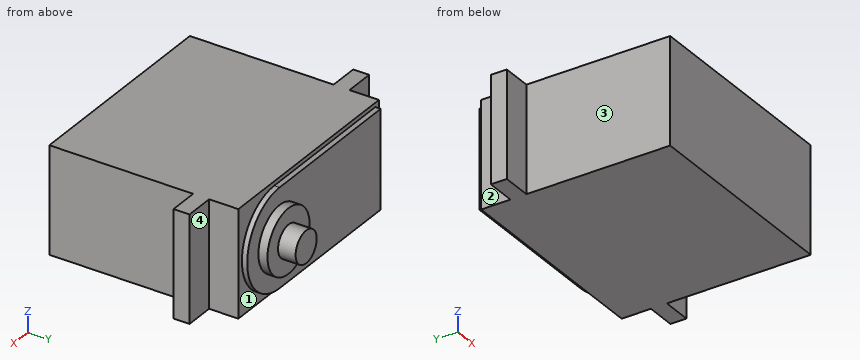
from build123d import *

# Parameters (mm, degrees)
RESSALTO_EXTRUS_O1_DEPTH = 10
RESSALTO_EXTRUS_O2_DEPTH = 1
ESBO_O4_R                = 3
RESSALTO_EXTRUS_O3_DEPTH = 5
ESBO_O5_R                = 6
RESSALTO_EXTRUS_O4_DEPTH = 1.7


with BuildPart() as part:
    # Esboço1 → Ressalto-extrusão1 (new body, symmetric)
    with BuildSketch(Plane.XY):
        Polygon((20, -0.767915455), (25.568877633, -0.767915455), (25.568877633, -3.767915455), (20, -3.767915455), (20, -30.767915455), (-20, -30.767915455), (-20, -3.767915455), (-25.568877633, -3.767915455), (-25.568877633, -0.767915455), (-20, -0.767915455), (-20, 4.732084545), (20, 4.732084545), align=None)
    extrude(amount=RESSALTO_EXTRUS_O1_DEPTH, both=True)

    # Esboço3 → Ressalto-extrusão2 (add)
    with BuildSketch(Plane(origin=(0, 4.732084545, 0), x_dir=(1, 0, 0), z_dir=(0, 1, 0))):
        with BuildLine():
            Line((-19, 9.2), (9.8, 9.2))
            ThreePointArc((9.8, 9.2), (19, 0), (9.8, -9.2))
            Line((9.8, -9.2), (-19, -9.2))
            Line((-19, -9.2), (-19, 9.2))
        make_face()
    extrude(amount=RESSALTO_EXTRUS_O2_DEPTH)

    # Esboço4 → Ressalto-extrusão3 (add)
    with BuildSketch(Plane(origin=(0, 5.732084545, 0), x_dir=(1, 0, 0), z_dir=(0, 1, 0))):
        with Locations((9.8, 0)):
            Circle(ESBO_O4_R)
    extrude(amount=RESSALTO_EXTRUS_O3_DEPTH)

    # Esboço5 → Ressalto-extrusão4 (add)
    with BuildSketch(Plane(origin=(0, 5.732084545, 0), x_dir=(1, 0, 0), z_dir=(0, 1, 0))):
        with Locations((9.8, 0)):
            Circle(ESBO_O5_R)
    extrude(amount=RESSALTO_EXTRUS_O4_DEPTH)


solid = part.part
Could you check a few things on this model? Use its own coordinates, in mm. Face numbers are marked on the shaded views. A direction names the side the tool comes from. Give positions to 0.01 mm unless a question says otherwise; leave off trailing zeros. Order: outer loops, then holes, each group sorted by start corner. A loop starts at its lowest first (then second) coordinate and runs counter-clockwise, first axis right, second up.
1. Will these pins go through, and if not, where does the flat tip stop? P1, Ø10, axis at x = -8, z = -2.5, coming from the +Y side; P2, Ø0.5, axis at x = -3.5, y = 5.5, coming from the +Z side; P3, Ø6, axis at y = 3, z = 0.5, coming from the -X side.
2. I need wall thicknesses on L1, parallel to Y at x = 2, z = 8.5; L2, parallel to X at y = -8, z = 6; L3, parallel to Y at x = 10, z = -3.5. Which ranges of each line are inside material? Lowest first, please.
3. Suppose I cut it at D-D (z = -7). List the corners of the cut face in (x, y) for me, plus the area to 3 significant figures.
4. Suppose I cut it at C-C (y = -27). List the corners of the cut face in (x, z) for me, plus the area to 3 significant figures.
5. Suppose I cut it at A-A (z = 0). List the corners of the cut face in (x, y) for me, plus the area to 3 significant figures.
6. For the marked faces 1, 2, 3 and 4, which set-ups out of +Z, -Z, +X, -X, +Y, -Y let a thin tool reach every point of the face, with its end or its side?
7. Suppose I cut it at B-B (x = -14.5). List the corners of the cut face in (y, z) for me.
Solved:
1. P1: stops at y = 5.73
1. P2: stops at z = 9.2
1. P3: stops at x = -20
2. L1: y = -30.77 to 5.73
2. L2: x = -20 to 20
2. L3: y = -30.77 to 7.43
3. outline: (-25.57, -3.77) - (-20, -3.77) - (-20, -30.77) - (20, -30.77) - (20, -3.77) - (25.57, -3.77) - (25.57, -0.77) - (20, -0.77) - (20, 4.73) - (15.77, 4.73) - (15.77, 5.73) - (-19, 5.73) - (-19, 4.73) - (-20, 4.73) - (-20, -0.77) - (-25.57, -0.77) - close
3. area: 1,490 mm2
4. outline: (-20, -10) - (20, -10) - (20, 10) - (-20, 10) - close
4. area: 800 mm2
5. outline: (-25.57, -3.77) - (-20, -3.77) - (-20, -30.77) - (20, -30.77) - (20, -3.77) - (25.57, -3.77) - (25.57, -0.77) - (20, -0.77) - (20, 4.73) - (19, 4.73) - (19, 5.73) - (15.8, 5.73) - (15.8, 7.43) - (12.8, 7.43) - (12.8, 10.73) - (6.8, 10.73) - (6.8, 7.43) - (3.8, 7.43) - (3.8, 5.73) - (-19, 5.73) - (-19, 4.73) - (-20, 4.73) - (-20, -0.77) - (-25.57, -0.77) - close
5. area: 1,530 mm2
6. face 1: +Y
6. face 2: +Z, -Z, -X, +Y
6. face 3: +Z, -Z, -X, -Y
6. face 4: +Z, -Z, +X, +Y
7. outline: (-30.77, -10) - (4.73, -10) - (4.73, -9.2) - (5.73, -9.2) - (5.73, 9.2) - (4.73, 9.2) - (4.73, 10) - (-30.77, 10) - close
